Source: CAD feature listing. Evaluate the final solid. Frame: model axes, mm. A direction names the side the tool comes from. Give positions to 0.01 mm unless a question says otherwise; leave off trailing zeros. Write each loop counter-clockwise with the first axis right and the second up, starting at its lowest first coordinate (ties: lowest second). Pieces come first, ordered by that corner, then holes.
```python
from build123d import *

# Parameters (mm, degrees)
F0_W     = 241.3
F0_H     = 114.3
F1_DEPTH = 12.7
F2_W     = 190.5
F2_H     = 63.5
F3_DEPTH = 12.7
F4_R     = 6.35
F5_DEPTH = 12.7


# Not quite as in the source:
# - a feature names something its author has since deleted; it is built from what else it names


with BuildPart() as f1:
    # F0 (on Top) → F1 (new body)
    with BuildSketch(Plane.XY):
        Rectangle(F0_W, F0_H)
    extrude(amount=F1_DEPTH)

    # F2 (on face) → F3 (join)
    with BuildSketch(Plane(origin=(0, 0, 0), x_dir=(1, 0, 0), z_dir=(0, 0, -1))):
        Rectangle(F2_W, F2_H)
    extrude(amount=F3_DEPTH)

    # F4 (on face) → F5 (cut)
    with BuildSketch(Plane.XY.offset(12.7)):
        with Locations((-107.95, 44.45)):
            Circle(F4_R)
        with Locations((-107.95, -44.45)):
            Circle(F4_R)
        with Locations((107.95, -44.45)):
            Circle(F4_R)
        with Locations((107.95, 44.45)):
            Circle(F4_R)
        with Locations((0, 44.45)):
            Circle(F4_R)
        with Locations((0, -44.45)):
            Circle(F4_R)
    extrude(amount=-F5_DEPTH, mode=Mode.SUBTRACT)


solid = f1.part
```
1. Line query: L1, parallel to Y at x = -107.95, z = 6.25; L2, parallel to X at y = -47, z = 4.5; L3, parallel to Y at x = -107, z = 7.5. Output: solid intervals per line, ascending.
2. Contact query for flat-ended pins moving along their axis: P1, Ø11.5, axis at x = -107.95, y = -44.45, coming from the +Z side; P2, Ø4, axis at x = -32.5, z = -6.5, coming from the +Y side; P3, Ø4, axis at y = -15, z = -5.5, coming from the +X side; P4, Ø10, axis at x = 46.5, z = -7, coming from the -Y side. Output: stop coordinate, or through.
3. Mould query, pull axis Y, two halves, no side actions, for faces 4 (the flat face through (-2, 1, 12.7)), 5 (the flat face through (-1, -31.75, -6)), 6 (the cylindrical face through (101.606, 44.729, 6.439)), 7 (the flat face through (-1, 31.75, -6)). Classes: +Y half, -Y half, draft (parallel to the pull), parting line (faces both ways), or undercut.
4. Cut plane D-D, the plane x = -43.5. Return the cut outline in (y, z), then the cut area to 3 significant figures.
5. Cut plane A-A, the plane z = 8.5. Return the cut outline in (x, y).
6. Cut plane B-B, the plane x = -107.95. Return the cut outline in (y, z).
7. Cut plane C-C, the plane y = -44.45. Return the cut outline in (x, z).
8. Access query for faces 1 (the cylindrical face through (-0.827, 50.746, 6.439)), 2 (the flat face through (-95.25, 0, -6)), 3 (the flat face through (95.25, 0, -6)). Directions: +Z, -Z, +X, -X, +Y, -Y. A direction counts if a zero-diameter tool reaches every point of the face in a straight line with its end or side. Return the directions, or none.
Response values:
1. L1: y = -57.15 to -50.8, -38.1 to 38.1, 50.8 to 57.15
1. L2: x = -120.65 to -113.77, -102.13 to -5.82, 5.82 to 102.13, 113.77 to 120.65
1. L3: y = -57.15 to -50.73, -38.17 to 38.17, 50.73 to 57.15
2. P1: passes through
2. P2: stops at y = 31.75
2. P3: stops at x = 95.25
2. P4: stops at y = -31.75
3. face 4: draft
3. face 5: -Y half
3. face 6: undercut
3. face 7: +Y half
4. outline: (-57.15, 0) - (-31.75, 0) - (-31.75, -12.7) - (31.75, -12.7) - (31.75, 0) - (57.15, 0) - (57.15, 12.7) - (-57.15, 12.7) - close
4. area: 2,260 mm2
5. outline: (-120.65, -57.15) - (120.65, -57.15) - (120.65, 57.15) - (-120.65, 57.15) - close; hole circle Ø12.7 at (-107.95, -44.45); hole circle Ø12.7 at (-107.95, 44.45); hole circle Ø12.7 at (0, -44.45); hole circle Ø12.7 at (0, 44.45); hole circle Ø12.7 at (107.95, -44.45); hole circle Ø12.7 at (107.95, 44.45)
6. outline: (-57.15, 0) - (-50.8, 0) - (-50.8, 12.7) - (-57.15, 12.7) - close; (-38.1, 0) - (38.1, 0) - (38.1, 12.7) - (-38.1, 12.7) - close; (50.8, 0) - (57.15, 0) - (57.15, 12.7) - (50.8, 12.7) - close
7. outline: (-120.65, 0) - (-114.3, 0) - (-114.3, 12.7) - (-120.65, 12.7) - close; (-101.6, 0) - (-6.35, 0) - (-6.35, 12.7) - (-101.6, 12.7) - close; (6.35, 0) - (101.6, 0) - (101.6, 12.7) - (6.35, 12.7) - close; (114.3, 0) - (120.65, 0) - (120.65, 12.7) - (114.3, 12.7) - close
8. face 1: +Z, -Z
8. face 2: -Z, -X, +Y, -Y
8. face 3: -Z, +X, +Y, -Y
